Can you work these out from the model? Positions are in its coordinate system, mm. A direction names the side the tool comes from. Give positions to 0.01 mm unless a question says otherwise; leave off trailing zeros. Loops run counter-clockwise (first coordinate to the right, second up) from the corner with the lowest first, then second, coordinate; pieces in that order, holes last. Notation, with made-up numbers: M 64.5,77 L 89.5,77 A31 cw 89.5,104 Z; hole C -13.75,-21 d4. An arc over 180 degrees is marked long. One line per item, written item: value. Start each with the question number.
from build123d import *

# Parameters (mm, degrees)
SKETCH1_R           = 30
SKETCH1_R_2         = 7
BOSS_EXTRUDE1_DEPTH = 10
FILLET1_R           = 10
FILLET3_R           = 10
CUT_EXTRUDE1_DEPTH  = 5
CUT_EXTRUDE3_START  = 10
SKETCH12_R          = 11.339564337
CUT_EXTRUDE3_DEPTH  = 21


with BuildPart() as part:
    # Sketch1 → Boss-Extrude1 (new body, symmetric)
    with BuildSketch(Plane.XY):
        with BuildLine():
            Line((128.063755469, 9.084385863), (27.935473676, 25.760615491))
            ThreePointArc((27.935473676, 25.760615491), (-38, 0), (27.935473676, -25.760615491))
            Line((27.935473676, -25.760615491), (128.063755469, -9.084385863))
            ThreePointArc((128.063755469, -9.084385863), (155, 0), (128.063755469, 9.084385863))
        make_face()
        Circle(SKETCH1_R, mode=Mode.SUBTRACT)
        with Locations((140, 0)):
            Circle(SKETCH1_R_2, mode=Mode.SUBTRACT)
    extrude(amount=BOSS_EXTRUDE1_DEPTH, both=True)

    # Fillet1
    fillet1_edges = [part.edges().sort_by_distance(p)[0] for p in [
        (27.935473676, -25.760615491, 0),
        (27.935473676, 25.760615491, 0),
    ]]
    fillet(fillet1_edges, radius=FILLET1_R)

    # Fillet3
    fillet3_edges = [part.edges().sort_by_distance(p)[0] for p in [
        (128.063755469, -9.084385863, 0),
        (128.063755469, 9.084385863, 0),
    ]]
    fillet(fillet3_edges, radius=FILLET3_R)

    # Sketch2 → Cut-Extrude1 (cut)
    with BuildSketch(Plane.XY.offset(10)):
        with BuildLine():
            Line((41.828554558, 17.870982725), (122.111301675, 4.5))
            ThreePointArc((122.111301675, 4.5), (126.611301675, 0), (122.111301675, -4.5))
            Line((122.111301675, -4.5), (41.828554558, -17.870982725))
            ThreePointArc((41.828554558, -17.870982725), (37.231968897, -16.217361812), (36.238855523, -11.43439331))
            ThreePointArc((36.238855523, -11.43439331), (38, 0), (36.238855523, 11.43439331))
            ThreePointArc((36.238855523, 11.43439331), (37.231968897, 16.217361812), (41.828554558, 17.870982725))
        make_face()
    cut_extrude1 = extrude(amount=-CUT_EXTRUDE1_DEPTH, mode=Mode.SUBTRACT)

    # Mirror1: Cut-Extrude1 across plane
    add(cut_extrude1.mirror(Plane.XY), mode=Mode.SUBTRACT)

    # Sketch12 → Cut-Extrude3 (cut, through all)
    with BuildSketch(Plane.XY.offset(CUT_EXTRUDE3_START)):
        with Locations((80.10699969, 0)):
            Circle(SKETCH12_R)
    extrude(amount=-CUT_EXTRUDE3_DEPTH, mode=Mode.SUBTRACT)


solid = part.part
Q1. I need wall thicknesses on line 1 along Y through (x, z) = (140, 3.5); line 2 along X through (y, z) = (1.5, 6); line 3 along X through (y, z) = (-8, 1.75). Which ranges of each line are inside material? Lowest first, please.
Q2. If we section it at D-D, the plane y = -21.5: Write out the boundary of the cut face in (x, z).
Q3. If we section it at C-C, the plane x = 140: Write out the boundary of the cut face in (y, z).
Q4. If we mould it in two halves opening along Y, with no side actions, what happens to faces 4 (the face through (134.84, 4.73, -0.14)), 5 (the face through (155, 0, 0)), 6 (the face through (28.36, 26.11, 0.14))? For each: released by +Y, released by -Y, zero draft, split by the parting line, or undercut.
Q5. If we section it at B-B, the plane z = -1.75: Write out the boundary of the cut face in (x, y), plus the area to 3 significant figures.
Q6. If we section it at A-A, the plane y = 0: Write out the boundary of the cut face in (x, z), plus the area to 3 significant figures.
Q7. For P1, Ø5, axis at y = -28.5, z = -3, coming from the +X side; P2, Ø12, axis at y = 17.5, z = -2, coming from the -X side; P3, Ø1.5, axis at x = 98.5, z = 1, coming from the +Y side; P4, Ø18, axis at x = 103, y = -2, coming from the +Z side, each with a flat end and sliding along its axis, tell me the tip position at first contact or that it passes through.
Q8. Which directions (+Z, -Z, +X, -X, +Y, -Y) give clear straight access to the entire face, cutting with the end or side of a thin tool? Please do faces 1 (the face through (38, 0, -8)), 2 (the face through (77.729, 17.468, 0.14)), 3 (the face through (37.186, 16.163, 7.535)).
Response:
1. line 1: -15 to -7, 7 to 15
1. line 2: -37.97 to -29.96, 29.96 to 37.97, 126.35 to 133.16, 146.84 to 154.92
1. line 3: -37.15 to -28.91, 28.91 to 72.07, 88.14 to 152.69
2. outline: M -31.33,-10 L -20.92,-10 L -20.92,10 L -31.33,10 Z; M 20.92,-10 L 53.52,-10 L 53.52,10 L 20.92,10 Z
3. outline: M -15,-10 L -7,-10 L -7,10 L -15,10 Z; M 7,-10 L 15,-10 L 15,10 L 7,10 Z
4. face 4: undercut
4. face 5: split by the parting line
4. face 6: released by +Y
5. outline: M 25.92,-27.79 A10 cw 31.1,-25.23 L 123.07,-9.92 A10 cw 130.83,-11.87 A15 ccw long 130.83,11.87 A10 cw 123.07,9.92 L 31.1,25.23 A10 cw 25.92,27.79 A38 ccw long Z; hole C 0,0 d60; hole C 80.11,0 d22.68; hole C 140,0 d14
5. area: 4,960 mm^2
6. outline: M -38,-10 L -30,-10 L -30,10 L -38,10 Z; M 30,-10 L 38,-10 L 38,-5 L 68.77,-5 L 68.77,5 L 38,5 L 38,10 L 30,10 Z; M 91.45,-5 L 126.61,-5 L 126.61,-10 L 133,-10 L 133,10 L 126.61,10 L 126.61,5 L 91.45,5 Z; M 147,-10 L 155,-10 L 155,10 L 147,10 Z
6. area: 1,270 mm^2
7. P1: x = 28.59
7. P2: x = -36.22
7. P3: y = 14.13
7. P4: z = 10
8. face 1: -Z
8. face 2: +Z, -Z, +Y
8. face 3: +Z
